from build123d import *

# Parameters (mm, degrees)
BOSS_EXTRUDE1_DEPTH      = 25.4
SKETCH2_R                = 12.7
BOSS_EXTRUDE2_DEPTH      = 50.8
SKETCH3_R                = 12.7
BOSS_EXTRUDE3_DEPTH      = 25.4
SKETCH4_W                = 6.35
SKETCH4_H                = 8.89
SKETCH4_W_2              = 3.81
SKETCH4_H_2              = 6.35
CUT_EXTRUDE1_DEPTH       = 2.54
SKETCH5_W                = 1.27
SKETCH5_H                = 10.16
CUT_EXTRUDE2_DEPTH       = 2.54
CUT_EXTRUDE3_DEPTH       = 2.54
CUT_EXTRUDE4_DEPTH       = 2.54
CUT_EXTRUDE5_DEPTH       = 2.54
CUT_EXTRUDE6_DEPTH       = 2.54
SKETCH11_W               = 6.35
SKETCH11_H               = 3.81
CUT_EXTRUDE7_DEPTH       = 8.464872704
CUT_EXTRUDE7_DEPTH_BACK  = 2.54
CUT_EXTRUDE8_DEPTH       = 2.54
SKETCH13_W               = 8.89
SKETCH13_H               = 11.43
SKETCH13_W_2             = 6.35
SKETCH13_H_2             = 3.81
CUT_EXTRUDE9_DEPTH       = 2.54
SKETCH14_W               = 6.35
SKETCH14_H               = 3.81
CUT_EXTRUDE10_DEPTH      = 1
CUT_EXTRUDE10_DEPTH_BACK = 2.54


with BuildPart() as part:
    # Sketch1 → Boss-Extrude1 (new body)
    with BuildSketch(Plane(origin=(0, 0, 0), x_dir=(0, 0, -1), z_dir=(1, 0, 0))):
        Polygon((0, 25.4), (-14.929745408, 20.549031657), (-24.156835514, 7.849031657), (-24.156835514, -7.849031657), (-14.929745408, -20.549031657), (0, -25.4), (14.929745408, -20.549031657), (24.156835514, -7.849031657), (24.156835514, 7.849031657), (14.929745408, 20.549031657), align=None)
    extrude(amount=BOSS_EXTRUDE1_DEPTH)

    # Sketch2 → Boss-Extrude2 (add)
    with BuildSketch(Plane(origin=(25.4, 0, 0), x_dir=(0, 0, -1), z_dir=(1, 0, 0))):
        Circle(SKETCH2_R)
    extrude(amount=BOSS_EXTRUDE2_DEPTH)

    # Sketch3 → Boss-Extrude3 (add)
    with BuildSketch(Plane.ZY):
        Circle(SKETCH3_R)
    extrude(amount=BOSS_EXTRUDE3_DEPTH)

    # Sketch4 → Cut-Extrude1 (cut)
    with BuildSketch(Plane(origin=(0, 14.199031657, 19.543290461), x_dir=(1, 0, 0), z_dir=(0, 0.587785252, 0.809016994))):
        with Locations((12.7, 0)):
            Rectangle(SKETCH4_W, SKETCH4_H)
        with Locations((12.7, 0)):
            Rectangle(SKETCH4_W_2, SKETCH4_H_2, mode=Mode.SUBTRACT)
    extrude(amount=-CUT_EXTRUDE1_DEPTH, mode=Mode.SUBTRACT)

    # Sketch5 → Cut-Extrude2 (cut)
    with BuildSketch(Plane(origin=(0, 22.974515829, 7.464872704), x_dir=(1, 0, 0), z_dir=(0, 0.951056516, 0.309016994))):
        with Locations((12.7, 0)):
            Rectangle(SKETCH5_W, SKETCH5_H)
    extrude(amount=-CUT_EXTRUDE2_DEPTH, mode=Mode.SUBTRACT)

    # Sketch6 → Cut-Extrude3 (cut)
    with BuildSketch(Plane(origin=(0, 22.974515829, -7.464872704), x_dir=(1, 0, 0), z_dir=(0, 0.951056516, -0.309016994))):
        Polygon((8.89, 3.175), (15.875, 3.175), (15.875, 0.635), (8.255, 0.635), (8.255, -4.445), (16.51, -4.445), (16.51, -3.175), (9.525, -3.175), (9.525, -0.635), (17.145, -0.635), (17.145, 4.445), (8.89, 4.445), align=None)
    extrude(amount=-CUT_EXTRUDE3_DEPTH, mode=Mode.SUBTRACT)

    # Sketch8 → Cut-Extrude4 (cut)
    with BuildSketch(Plane(origin=(0, 14.199031657, -19.543290461), x_dir=(-1, 0, 0), z_dir=(0, 0.587785252, -0.809016994))):
        Polygon((-8.89, -5.715), (-8.89, -4.445), (-15.875, -4.445), (-15.875, -0.635), (-8.89, -0.635), (-8.89, 0.635), (-15.875, 0.635), (-15.875, 4.445), (-8.89, 4.445), (-8.89, 5.715), (-17.145, 5.715), (-17.145, -5.715), align=None)
    extrude(amount=-CUT_EXTRUDE4_DEPTH, mode=Mode.SUBTRACT)

    # Sketch9 → Cut-Extrude5 (cut)
    with BuildSketch(Plane(origin=(0, 0, -24.156835514), x_dir=(-1, 0, 0), z_dir=(0, 0, -1))):
        Polygon((-9.525, -5.08), (-8.255, -5.08), (-8.255, 0.635), (-15.875, 0.635), (-15.875, 5.08), (-17.145, 5.08), (-17.145, -5.08), (-15.875, -5.08), (-15.875, -0.635), (-9.525, -0.635), align=None)
    extrude(amount=-CUT_EXTRUDE5_DEPTH, mode=Mode.SUBTRACT)

    # Sketch10 → Cut-Extrude6 (cut)
    with BuildSketch(Plane(origin=(0, -14.199031657, -19.543290461), x_dir=(-1, 0, 0), z_dir=(0, -0.587785252, -0.809016994))):
        Polygon((-8.89, 5.715), (-17.145, 5.715), (-17.145, -0.635), (-9.525, -0.635), (-9.525, -4.445), (-16.51, -4.445), (-16.51, -5.715), (-8.255, -5.715), (-8.255, 0.635), (-15.875, 0.635), (-15.875, 4.445), (-8.89, 4.445), align=None)
    extrude(amount=-CUT_EXTRUDE6_DEPTH, mode=Mode.SUBTRACT)

    # Sketch11 → Cut-Extrude7 (cut, two sides)
    with BuildSketch(Plane(origin=(0, -22.974515829, -7.464872704), x_dir=(1, 0, 0), z_dir=(0, -0.951056516, -0.309016994))) as cut_extrude7_sk:
        Polygon((17.145, 0.635), (9.525, 0.635), (9.525, 4.445), (16.51, 4.445), (16.51, 5.715), (8.255, 5.715), (8.255, -5.715), (17.145, -5.715), align=None)
        with Locations((12.7, -2.54)):
            Rectangle(SKETCH11_W, SKETCH11_H, mode=Mode.SUBTRACT)
    extrude(amount=CUT_EXTRUDE7_DEPTH, mode=Mode.SUBTRACT)
    extrude(cut_extrude7_sk.sketch, amount=-CUT_EXTRUDE7_DEPTH_BACK, mode=Mode.SUBTRACT)

    # Sketch12 → Cut-Extrude8 (cut)
    with BuildSketch(Plane(origin=(0, -22.974515829, 7.464872704), x_dir=(1, 0, 0), z_dir=(0, -0.951056516, 0.309016994))):
        Polygon((8.89, 4.445), (15.875, 4.445), (15.875, -5.08), (17.145, -5.08), (17.145, 5.715), (8.89, 5.715), align=None)
    extrude(amount=-CUT_EXTRUDE8_DEPTH, mode=Mode.SUBTRACT)

    # Sketch13 → Cut-Extrude9 (cut)
    with BuildSketch(Plane(origin=(0, -14.199031657, 19.543290461), x_dir=(1, 0, 0), z_dir=(0, -0.587785252, 0.809016994))):
        with Locations((12.7, 0)):
            Rectangle(SKETCH13_W, SKETCH13_H)
        with Locations((12.7, -2.54)):
            Rectangle(SKETCH13_W_2, SKETCH13_H_2, mode=Mode.SUBTRACT)
        with Locations((12.7, 2.54)):
            Rectangle(SKETCH13_W_2, SKETCH13_H_2, mode=Mode.SUBTRACT)
    extrude(amount=-CUT_EXTRUDE9_DEPTH, mode=Mode.SUBTRACT)

    # Sketch14 → Cut-Extrude10 (cut, two sides)
    with BuildSketch(Plane.XY.offset(24.156835514)) as cut_extrude10_sk:
        Polygon((15.875, -0.635), (15.875, -5.08), (17.145, -5.08), (17.145, 5.715), (8.255, 5.715), (8.255, -0.635), align=None)
        with Locations((12.7, 2.54)):
            Rectangle(SKETCH14_W, SKETCH14_H, mode=Mode.SUBTRACT)
    extrude(amount=CUT_EXTRUDE10_DEPTH, mode=Mode.SUBTRACT)
    extrude(cut_extrude10_sk.sketch, amount=-CUT_EXTRUDE10_DEPTH_BACK, mode=Mode.SUBTRACT)


solid = part.part
Source: CAD feature listing. Evaluate the final solid. Frame: model axes, mm. A direction names the side the tool comes from. Round coordinates to 2 decimals unless told otherwise and drop trailing zeros. Loops run counter-clockwise (first coordinate to the right, second up) from the corner with the lowest first, then second, coordinate; pieces in that order, holes last.
Q1. Section A-A, the plane x = 50. Return loops of the section in (y, z).
Q2. Section B-B, the plane y = -3. Return loops of the section in (x, z) (3 decimals).
Q3. Ray query, line 1 (X direction, y = -20.5, z = -3); line 2 (Z direction, x = 62.5, y = -3.5); line 3 (Z direction, x = 45, y = -11). Return the intervals inside material, ascending.
Q4. First-contact query: P1, Ø1.7, axis at y = 14.5, z = 18.5, coming from the +X side; P2, Ø5, axis at x = 61, z = 16.5, coming from the -Y side; P3, Ø1.3, axis at y = 2.5, z = 23, coming from the -X side; P4, Ø10, axis at x = 7.5, z = 17.5, coming from the +Y side. Flat tips, straight axial feed; report the tip coordinate or a pass-through.
Q5. Access query for faces 1 (the face through (15.875, 3, 23)), 2 (the face through (0, 12, 6)), 3 (the face through (13, -0.635, -23)), 4 (the face through (16.51, -23, -2)). Directions: +Z, -Z, +X, -X, +Y, -Y. A direction counts if a zero-diameter tool reaches every point of the face in a straight line with its end or side. Return the directions, or none.
Q6. Mould query, pull axis Y, two halves, no side actions, for faces 5 (the face through (13.066, 22.765, -4.058)), 6 (the face through (9.525, -23, -5)), 7 (the face through (12.638, -12.641, 17.535)), 8 (the face through (8.255, -2, -23)). Classes: pulls with the +Y half, pulls with the -Y half, needs draft (parallel to the pull), parting line crosses it, or undercut.
Solutions:
1. outline: circle Ø25.4 at (0, 0)
2. outline: (-25.4, -12.341) - (0, -12.341) - (0, -24.157) - (8.255, -24.157) - (8.255, -21.617) - (9.525, -21.617) - (9.525, -24.157) - (15.875, -24.157) - (15.875, -21.617) - (17.145, -21.617) - (17.145, -24.157) - (25.4, -24.157) - (25.4, -12.341) - (76.2, -12.341) - (76.2, 12.341) - (25.4, 12.341) - (25.4, 24.157) - (17.145, 24.157) - (17.145, 21.617) - (15.875, 21.617) - (15.875, 24.157) - (0, 24.157) - (0, 12.341) - (-25.4, 12.341) - close
3. line 1: x = 0 to 25.4
3. line 2: z = -12.21 to 12.21
3. line 3: z = -6.35 to 6.35
4. P1: stops at x = 25.4
4. P2: passes through
4. P3: stops at x = 0
4. P4: stops at y = 21.34
5. face 1: +Z
5. face 2: -X
5. face 3: -Z
5. face 4: none
6. face 5: pulls with the +Y half
6. face 6: needs draft
6. face 7: undercut
6. face 8: undercut
